Could you check a few things on this model? Use its own coordinates, in mm. Face numbers are marked on the shaded views. A direction names the side the tool comes from. Give positions to 0.01 mm unless a question says otherwise; leave off trailing zeros. Write each loop counter-clockwise with the first axis right and the second up, starting at its lowest first coordinate (ties: lowest second). Pieces come first, ordered by that corner, then holes. Notation, with made-up numbers: (71, -13.75) -> (121, -13.75) arc R24 ccw to (121, 1.25) -> close; hole circle Ø5 at (-32.75, 84.25). An arc over 180 degrees is marked (long way). Write item = value, one per line. Start each with the question number.
```python
from build123d import *

# Parameters (mm, degrees)
F0_R     = 3
F1_DEPTH = 20


with BuildPart() as f1:
    # F0 (on Front) → F1 (new body)
    with BuildSketch(Plane.XZ):
        with BuildLine():
            Line((-13.020127, 8), (-16, 8))
            ThreePointArc((-16, 8), (-24, 0), (-16, -8))
            Line((-16, -8), (16, -8))
            ThreePointArc((16, -8), (24, 0), (16, 8))
            Line((16, 8), (6.979873, 8))
            Line((6.979873, 8), (6.979873, 16))
            Line((6.979873, 16), (-13.020127, 16))
            Line((-13.020127, 16), (-13.020127, 8))
        make_face()
        with Locations((-16, 0)):
            Circle(F0_R, mode=Mode.SUBTRACT)
        with Locations((16, 0)):
            Circle(F0_R, mode=Mode.SUBTRACT)
    extrude(amount=F1_DEPTH)


solid = f1.part
```
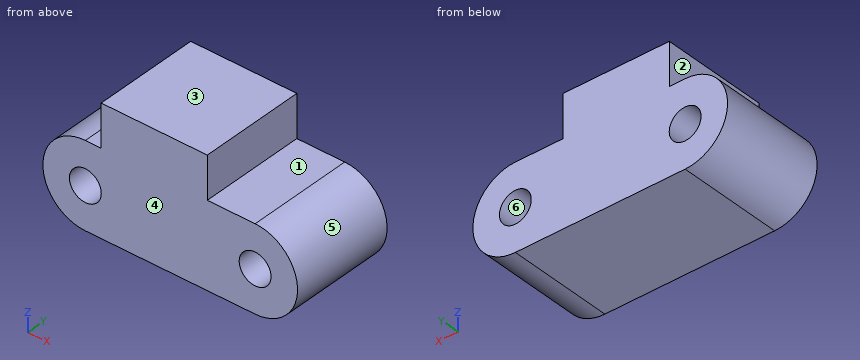
(1) We'd pull the mould along Z, two halves only. Please class the marked faces 4, 5 and 6: released by +Z, released by -Z, zero draft, split by the parting line, or undercut.
(2) Imagine slicing it at B-B (z = 0). Please give me the cut outline in (x, y).
(3) On a 3-axis mill with a long thin cutter (end or side, diameter ignored), from which of +Z, -Z, +X, -X, +Y, -Y can I reach the whole of each face in a straight line? I mean the marked faces 1, 2 and 3. Say none if no direction works.
(4) Imagine slicing it at D-D (x = 11). Please give me the cut outline in (y, z).
(5) I'm going to push flat-ended pins straight in: pin 1 (2.5 mm diameter, centred on y = -9.5, z = 11, fed in from +X); pin 2 (6 mm diameter, centred on x = 15.5, z = 12, fed in from -Y); pin 3 (2.5 mm diameter, centred on x = 9.5, y = -8, fed in from +Z); pin 4 (10 mm diameter, centred on y = -2.5, z = -5.5, fed in from +X). Where does each tip first touch, or does it pass through?
(6) If I drill on line 1 along Z through (x, y) = (-16, -9.25); line 2 along X through (y, z) = (-7.5, 0.5); line 3 along Z through (x, y) = (15, -9.75), over which ranges is the centre line in solid material (lowest first)? Write a range as from..to.
(7) Imagine slicing it at C-C (z = 13.5). Please give me the cut outline in (x, y), then the cut area to 3 significant figures.
(8) Imagine slicing it at A-A (y = -12). Please give me the cut outline in (x, z).
Answers below:
q1.face_4 = zero draft
q1.face_5 = split by the parting line
q1.face_6 = undercut
q2.outline = (-24, -20) -> (-19, -20) -> (-19, 0) -> (-24, 0) -> close; (-13, -20) -> (13, -20) -> (13, 0) -> (-13, 0) -> close; (19, -20) -> (24, -20) -> (24, 0) -> (19, 0) -> close
q3.face_1 = +Z, +X, +Y, -Y
q3.face_2 = +Z, -X, +Y, -Y
q3.face_3 = +Z, +X, -X, +Y, -Y
q4.outline = (-20, -8) -> (0, -8) -> (0, 8) -> (-20, 8) -> close
q5.pin_1 = 6.98
q5.pin_2 = through
q5.pin_3 = 8
q5.pin_4 = 23.98
q6.line_1 = -8..-3, 3..8
q6.line_2 = -23.98..-18.96, -13.04..13.04, 18.96..23.98
q6.line_3 = -8..-2.83, 2.83..8
q7.outline = (-13.02, -20) -> (6.98, -20) -> (6.98, 0) -> (-13.02, 0) -> close
q7.area = 400 mm^2
q8.outline = (-16, -8) -> (16, -8) arc R8 ccw to (16, 8) -> (6.98, 8) -> (6.98, 16) -> (-13.02, 16) -> (-13.02, 8) -> (-16, 8) arc R8 ccw to start; hole circle Ø6 at (-16, 0); hole circle Ø6 at (16, 0)
